Input: part model. Units: mm. Frame: model coordinates. Face numbers are marked on the shaded views. Round coordinates to 2 decimals unless told otherwise and drop trailing zeros. Write each loop counter-clockwise with the first axis right and the second up, starting at its lowest first coordinate (ties: lowest second). Pieces come first, ordered by that corner, then holes. Notation, with made-up numbers: (-7.5, -21) - (-3.5, -21) arc R38 cw to (-3.5, 17) - close; hole circle Ø6 at (9, -4.5). An arc over 180 degrees is marked (long way). One line per item, written item: value. Start each with the question number.
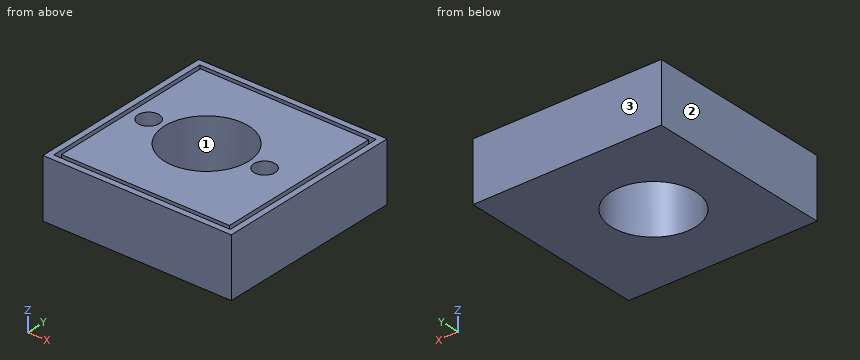
```python
from build123d import *

# Parameters (mm, degrees)
SKETCH2_W           = 112
SKETCH2_H           = 112
SKETCH2_R           = 25
BOSS_EXTRUDE1_DEPTH = 15
SKETCH3_W           = 112
SKETCH3_H           = 112
SKETCH3_W_2         = 105
SKETCH3_H_2         = 105
SKETCH3_W_3         = 100
SKETCH3_H_3         = 100
SKETCH3_R           = 6.35
SKETCH3_R_2         = 25
BOSS_EXTRUDE2_DEPTH = 20


with BuildPart() as part:
    # Sketch2 → Boss-Extrude1 (new body)
    with BuildSketch(Plane.XY):
        Rectangle(SKETCH2_W, SKETCH2_H)
        with Locations((-5, 0)):
            Circle(SKETCH2_R, mode=Mode.SUBTRACT)
    extrude(amount=BOSS_EXTRUDE1_DEPTH)

    # Sketch3 → Boss-Extrude2 (add)
    # profile 1 of 2: a face of its own
    with BuildSketch(Plane.XY.offset(15)):
        Rectangle(SKETCH3_W, SKETCH3_H)
        Rectangle(SKETCH3_W_2, SKETCH3_H_2, mode=Mode.SUBTRACT)
    # profile 2 of 2: a face of its own
    with BuildSketch(Plane.XY.offset(15)):
        Rectangle(SKETCH3_W_3, SKETCH3_H_3)
        with Locations((-39.5, 0)):
            Circle(SKETCH3_R, mode=Mode.SUBTRACT)
        with Locations((-5, 0)):
            Circle(SKETCH3_R_2, mode=Mode.SUBTRACT)
        with Locations((29.5, 0)):
            Circle(SKETCH3_R, mode=Mode.SUBTRACT)
    extrude(amount=BOSS_EXTRUDE2_DEPTH)


solid = part.part
```
Q1. Cut plane B-B, the plane y = 0. Output: boundary loops of the cut face in (x, z).
Q2. Cut plane D-D, the plane y = 44. Output: boundary loops of the cut face in (x, z), and give its area (3 significant figures).
Q3. Cut plane A-A, the plane z = 25. Output: boundary loops of the cut face in (x, y), and give its area (3 significant figures).
Q4. Pull-direction query (X, two-part tool) for the marked faces 1, 2 and 3; classes: pulls with the +X half, pulls with the -X half, needs draft (parallel to the pull), parting line crosses it, or undercut.
Q5. Cut plane C-C, the plane x = -5. Output: boundary loops of the cut face in (y, z).
Q6. Material intervals for probe 1 along Y at (x, z) = (29, 30); probe 2 along Y at (x, z) = (-5, 16); probe 3 along X at (y, z) = (-45.5, 31), sorted ascending. Write a range as from..to.
Q7. Contact query for a flat-ended pin moving along its axis: pin 1 Ø11.5 at (x, y) = (-39.5, 0) entering from +Z. Output: stop coordinate, or through.
A:
1. outline: (-56, 0) - (-30, 0) - (-30, 35) - (-33.15, 35) - (-33.15, 15) - (-45.85, 15) - (-45.85, 35) - (-50, 35) - (-50, 15) - (-52.5, 15) - (-52.5, 35) - (-56, 35) - close; (20, 0) - (56, 0) - (56, 35) - (52.5, 35) - (52.5, 15) - (50, 15) - (50, 35) - (35.85, 35) - (35.85, 15) - (23.15, 15) - (23.15, 35) - (20, 35) - close
2. outline: (-56, 0) - (56, 0) - (56, 35) - (52.5, 35) - (52.5, 15) - (50, 15) - (50, 35) - (-50, 35) - (-50, 15) - (-52.5, 15) - (-52.5, 35) - (-56, 35) - close
2. area: 3,820 mm²
3. outline: (-56, -56) - (56, -56) - (56, 56) - (-56, 56) - close; (-50, -50) - (50, -50) - (50, 50) - (-50, 50) - close; hole (-52.5, -52.5) - (52.5, -52.5) - (52.5, 52.5) - (-52.5, 52.5) - close; hole circle Ø12.7 at (-39.5, 0); hole circle Ø50 at (-5, 0); hole circle Ø12.7 at (29.5, 0)
3. area: 9,300 mm²
4. face 1: undercut
4. face 2: pulls with the -X half
4. face 3: needs draft
5. outline: (-56, 0) - (-25, 0) - (-25, 35) - (-50, 35) - (-50, 15) - (-52.5, 15) - (-52.5, 35) - (-56, 35) - close; (25, 0) - (56, 0) - (56, 35) - (52.5, 35) - (52.5, 15) - (50, 15) - (50, 35) - (25, 35) - close
6. probe 1: y = -56..-52.5, -50..-6.33, 6.33..50, 52.5..56
6. probe 2: y = -56..-52.5, -50..-25, 25..50, 52.5..56
6. probe 3: x = -56..-52.5, -50..50, 52.5..56
7. pin 1: stops at z = 15
